```python
from build123d import *

# Parameters (mm, degrees)
SKETCH1_W                    = 28.1256
SKETCH1_H                    = 33.5
SKETCH1_W_2                  = 15.5256
SKETCH1_H_2                  = 15
BASE_FLANGE2_DEPTH           = 0.8128
EDGE_FLANGE3_STRIP_W         = 4.7244
EDGE_FLANGE3_STRIP_H         = 0.8128
EDGE_FLANGE3_STRIP_CUT_DEPTH = 33.5
EDGE_FLANGE3_DEPTH           = 33.5
EDGE_FLANGE3_FLAT_DEPTH      = 0.8128
EDGE_FLANGE4_START           = 0.7366
EDGE_FLANGE4_DEPTH           = 56.7698
EDGE_FLANGE4_START_2         = 57.1
EDGE_FLANGE4_2_DEPTH         = 0.4064
EDGE_FLANGE4_3_DEPTH         = 56.3634
CUT_EXTRUDE1_REACH           = 94.079
SKETCH22_R                   = 2.05
CUT_EXTRUDE2_REACH           = 89.705
SKETCH23_W                   = 11.2634
SKETCH23_H                   = 10
CUT_EXTRUDE3_REACH           = 93.47


# Read off the part's stored shape, not the designer's step: Edge-Flange4
# Sheet-metal steps are written as plain solids
with BuildPart() as part:
    # Sketch1 → Base-Flange2 (new body)
    with BuildSketch(Plane.XY):
        Rectangle(SKETCH1_W, SKETCH1_H)
        with Locations((0, 0.59)):
            Rectangle(SKETCH1_W_2, SKETCH1_H_2, mode=Mode.SUBTRACT)
    extrude(amount=-BASE_FLANGE2_DEPTH)

    # Edge-Flange3 strip (across the edge) → Edge-Flange3 strip cut (cut)
    with BuildSketch(Plane(origin=(-14.0628, 16.75, 0), x_dir=(1, 0, 0), z_dir=(0, -1, 0))):
        with Locations((-0.8128, -0.4064)):
            Rectangle(EDGE_FLANGE3_STRIP_W, EDGE_FLANGE3_STRIP_H)
    extrude(amount=EDGE_FLANGE3_STRIP_CUT_DEPTH, mode=Mode.SUBTRACT)

    # Edge-Flange3 bend section (across the edge) → Edge-Flange3 (add)
    with BuildSketch(Plane(origin=(-14.0628, 16.75, 0), x_dir=(1, 0, 0), z_dir=(0, -1, 0))):
        with BuildLine():
            Line((0, 0.7366), (0.8128, 0.7366))
            ThreePointArc((0.8128, 0.7366), (1.028545145, 0.215745145), (1.5494, 0))
            Line((1.5494, 0), (1.5494, -0.8128))
            ThreePointArc((1.5494, -0.8128), (0.453808753, -0.358991247), (0, 0.7366))
        make_face()
    extrude(amount=EDGE_FLANGE3_DEPTH)

    # Edge-Flange3 profile (on flange) → Edge-Flange3 flat (add)
    with BuildSketch(Plane(origin=(-14.0628, 0, 0), x_dir=(0, -1, 0), z_dir=(-1, 0, 0))):
        Polygon((-16.75, 0.7366), (16.75, 0.7366), (16.75, 57.1), (41.75, 57.1), (41.75, 77.1), (-16.75, 77.1), align=None)
    extrude(amount=-EDGE_FLANGE3_FLAT_DEPTH)

    # Edge-Flange4 outline → Edge-Flange4 (cut)
    with BuildSketch(Plane.XY.offset(EDGE_FLANGE4_START)):
        with BuildLine():
            ThreePointArc((-13.25, -15.2006), (-13.468624211, -15.994121367), (-14.0628, -16.563707039))
            Line((-14.0628, -16.563707039), (-14.0628, -16.75))
            Line((-14.0628, -16.75), (-13.25, -16.75))
            Line((-13.25, -16.75), (-13.25, -15.2006))
        make_face()
    extrude(amount=EDGE_FLANGE4_DEPTH, mode=Mode.SUBTRACT)

    # Edge-Flange4 2 outline → Edge-Flange4 2 (cut)
    with BuildSketch(Plane.XY.offset(EDGE_FLANGE4_START_2)):
        with BuildLine():
            Line((-14.0628, -14.7942), (-14.0628, -16.563707039))
            ThreePointArc((-14.0628, -16.563707039), (-13.468624211, -15.994121367), (-13.25, -15.2006))
            Line((-13.25, -15.2006), (-13.25, -14.7942))
            Line((-13.25, -14.7942), (-14.0628, -14.7942))
        make_face()
    extrude(amount=EDGE_FLANGE4_2_DEPTH, mode=Mode.SUBTRACT)

    # Edge-Flange4 3 outline → Edge-Flange4 3 (add)
    with BuildSketch(Plane.XY.offset(EDGE_FLANGE4_START)):
        with BuildLine():
            Line((-26.0628, -16.75), (-14.7994, -16.75))
            ThreePointArc((-14.7994, -16.75), (-14.419503755, -16.702704924), (-14.0628, -16.563707039))
            Line((-14.0628, -16.563707039), (-14.0628, -15.2006))
            ThreePointArc((-14.0628, -15.2006), (-14.278545145, -15.721454855), (-14.7994, -15.9372))
            Line((-14.7994, -15.9372), (-26.0628, -15.9372))
            Line((-26.0628, -15.9372), (-26.0628, -16.75))
        make_face()
    extrude(amount=EDGE_FLANGE4_3_DEPTH)

    # Sketch22 → Cut-Extrude1 (cut, up to next)
    with BuildSketch(Plane.ZY.offset(14.0628), mode=Mode.PRIVATE) as cut_extrude1_sk1:
        with Locations((67.1, -31.91)):
            Circle(SKETCH22_R)
    cut_extrude1_tool1 = extrude(cut_extrude1_sk1.sketch, amount=-CUT_EXTRUDE1_REACH, mode=Mode.PRIVATE) & part.part
    # Sketch22 → Cut-Extrude1 (cut, up to next)
    with BuildSketch(Plane.ZY.offset(14.0628), mode=Mode.PRIVATE) as cut_extrude1_sk2:
        with Locations((67.1, -9.41)):
            Circle(SKETCH22_R)
    cut_extrude1_tool2 = extrude(cut_extrude1_sk2.sketch, amount=-CUT_EXTRUDE1_REACH, mode=Mode.PRIVATE) & part.part
    # Sketch22 → Cut-Extrude1 (cut, up to next)
    with BuildSketch(Plane.ZY.offset(14.0628), mode=Mode.PRIVATE) as cut_extrude1_sk3:
        with Locations((49.895058849, 0.59)):
            Circle(SKETCH22_R)
    cut_extrude1_tool3 = extrude(cut_extrude1_sk3.sketch, amount=-CUT_EXTRUDE1_REACH, mode=Mode.PRIVATE) & part.part
    # Sketch22 → Cut-Extrude1 (cut, up to next)
    with BuildSketch(Plane.ZY.offset(14.0628), mode=Mode.PRIVATE) as cut_extrude1_sk4:
        with Locations((29.995058849, 0.59)):
            Circle(SKETCH22_R)
    cut_extrude1_tool4 = extrude(cut_extrude1_sk4.sketch, amount=-CUT_EXTRUDE1_REACH, mode=Mode.PRIVATE) & part.part
    # Sketch22 → Cut-Extrude1 (cut, up to next)
    with BuildSketch(Plane.ZY.offset(14.0628), mode=Mode.PRIVATE) as cut_extrude1_sk5:
        with Locations((10.095058849, 0.59)):
            Circle(SKETCH22_R)
    cut_extrude1_tool5 = extrude(cut_extrude1_sk5.sketch, amount=-CUT_EXTRUDE1_REACH, mode=Mode.PRIVATE) & part.part
    add(cut_extrude1_tool1.solids().sort_by_distance((-14.0628, -31.91, 67.1))[0], mode=Mode.SUBTRACT)
    add(cut_extrude1_tool2.solids().sort_by_distance((-14.0628, -9.41, 67.1))[0], mode=Mode.SUBTRACT)
    add(cut_extrude1_tool3.solids().sort_by_distance((-14.0628, 0.59, 49.895059))[0], mode=Mode.SUBTRACT)
    add(cut_extrude1_tool4.solids().sort_by_distance((-14.0628, 0.59, 29.995059))[0], mode=Mode.SUBTRACT)
    add(cut_extrude1_tool5.solids().sort_by_distance((-14.0628, 0.59, 10.095059))[0], mode=Mode.SUBTRACT)

    # Sketch23 → Cut-Extrude2 (cut, up to next)
    with BuildSketch(Plane(origin=(0, -15.9372, 0), x_dir=(1, 0, 0), z_dir=(0, 1, 0)), mode=Mode.PRIVATE) as cut_extrude2_sk1:
        with Locations((-20.4311, -29.2366)):
            Rectangle(SKETCH23_W, SKETCH23_H)
    cut_extrude2_tool1 = extrude(cut_extrude2_sk1.sketch, amount=-CUT_EXTRUDE2_REACH, mode=Mode.PRIVATE) & part.part
    # Sketch23 → Cut-Extrude2 (cut, up to next)
    with BuildSketch(Plane(origin=(0, -15.9372, 0), x_dir=(1, 0, 0), z_dir=(0, 1, 0)), mode=Mode.PRIVATE) as cut_extrude2_sk2:
        with BuildLine():
            Line((-22.8128, -18.4866), (-22.8128, -10.4866))
            ThreePointArc((-22.8128, -10.4866), (-20.0628, -7.7366), (-17.3128, -10.4866))
            Line((-17.3128, -10.4866), (-17.3128, -18.4866))
            ThreePointArc((-17.3128, -18.4866), (-20.0628, -21.2366), (-22.8128, -18.4866))
        make_face()
    cut_extrude2_tool2 = extrude(cut_extrude2_sk2.sketch, amount=-CUT_EXTRUDE2_REACH, mode=Mode.PRIVATE) & part.part
    # Sketch23 → Cut-Extrude2 (cut, up to next)
    with BuildSketch(Plane(origin=(0, -15.9372, 0), x_dir=(1, 0, 0), z_dir=(0, 1, 0)), mode=Mode.PRIVATE) as cut_extrude2_sk3:
        with BuildLine():
            Line((-22.8128, -39.9866), (-22.8128, -47.9866))
            ThreePointArc((-22.8128, -47.9866), (-20.0628, -50.7366), (-17.3128, -47.9866))
            Line((-17.3128, -47.9866), (-17.3128, -39.9866))
            ThreePointArc((-17.3128, -39.9866), (-20.0628, -37.2366), (-22.8128, -39.9866))
        make_face()
    cut_extrude2_tool3 = extrude(cut_extrude2_sk3.sketch, amount=-CUT_EXTRUDE2_REACH, mode=Mode.PRIVATE) & part.part
    add(cut_extrude2_tool1.solids().sort_by_distance((-20.4311, -15.9372, 29.2366))[0], mode=Mode.SUBTRACT)
    add(cut_extrude2_tool2.solids().sort_by_distance((-20.0628, -15.9372, 14.4866))[0], mode=Mode.SUBTRACT)
    add(cut_extrude2_tool3.solids().sort_by_distance((-20.0628, -15.9372, 43.9866))[0], mode=Mode.SUBTRACT)

    # Sketch26 → Cut-Extrude3 (cut, up to next)
    with BuildSketch(Plane.XY, mode=Mode.PRIVATE) as cut_extrude3_sk1:
        with BuildLine():
            Line((8.8128, -13.75), (10.3128, -13.75))
            ThreePointArc((10.3128, -13.75), (11.6128, -12.45), (10.3128, -11.15))
            Line((10.3128, -11.15), (8.8128, -11.15))
            ThreePointArc((8.8128, -11.15), (7.5128, -12.45), (8.8128, -13.75))
        make_face()
    cut_extrude3_tool1 = extrude(cut_extrude3_sk1.sketch, amount=-CUT_EXTRUDE3_REACH, mode=Mode.PRIVATE) & part.part
    # Sketch26 → Cut-Extrude3 (cut, up to next)
    with BuildSketch(Plane.XY, mode=Mode.PRIVATE) as cut_extrude3_sk2:
        with BuildLine():
            Line((-8.7634, -13.75), (-7.2634, -13.75))
            ThreePointArc((-7.2634, -13.75), (-5.9634, -12.45), (-7.2634, -11.15))
            Line((-7.2634, -11.15), (-8.7634, -11.15))
            ThreePointArc((-8.7634, -11.15), (-10.0634, -12.45), (-8.7634, -13.75))
        make_face()
    cut_extrude3_tool2 = extrude(cut_extrude3_sk2.sketch, amount=-CUT_EXTRUDE3_REACH, mode=Mode.PRIVATE) & part.part
    # Sketch26 → Cut-Extrude3 (cut, up to next)
    with BuildSketch(Plane.XY, mode=Mode.PRIVATE) as cut_extrude3_sk3:
        with BuildLine():
            Line((8.8128, 11.45), (10.3128, 11.45))
            ThreePointArc((10.3128, 11.45), (11.6128, 12.75), (10.3128, 14.05))
            Line((10.3128, 14.05), (8.8128, 14.05))
            ThreePointArc((8.8128, 14.05), (7.5128, 12.75), (8.8128, 11.45))
        make_face()
    cut_extrude3_tool3 = extrude(cut_extrude3_sk3.sketch, amount=-CUT_EXTRUDE3_REACH, mode=Mode.PRIVATE) & part.part
    # Sketch26 → Cut-Extrude3 (cut, up to next)
    with BuildSketch(Plane.XY, mode=Mode.PRIVATE) as cut_extrude3_sk4:
        with BuildLine():
            Line((-8.7634, 11.45), (-7.2634, 11.45))
            ThreePointArc((-7.2634, 11.45), (-5.9634, 12.75), (-7.2634, 14.05))
            Line((-7.2634, 14.05), (-8.7634, 14.05))
            ThreePointArc((-8.7634, 14.05), (-10.0634, 12.75), (-8.7634, 11.45))
        make_face()
    cut_extrude3_tool4 = extrude(cut_extrude3_sk4.sketch, amount=-CUT_EXTRUDE3_REACH, mode=Mode.PRIVATE) & part.part
    add(cut_extrude3_tool1.solids().sort_by_distance((9.5628, -12.45, 0))[0], mode=Mode.SUBTRACT)
    add(cut_extrude3_tool2.solids().sort_by_distance((-8.0134, -12.45, 0))[0], mode=Mode.SUBTRACT)
    add(cut_extrude3_tool3.solids().sort_by_distance((9.5628, 12.75, 0))[0], mode=Mode.SUBTRACT)
    add(cut_extrude3_tool4.solids().sort_by_distance((-8.0134, 12.75, 0))[0], mode=Mode.SUBTRACT)


solid = part.part
```
For this review, take the finished solid that the model builds, in its own axes (mm). A direction names the side the tool comes from. Coordinates: 2 decimals unless noted, no trailing zeros. Order: outer loops, then holes, each group sorted by start corner. A loop starts at its lowest first (then second) coordinate and runs counter-clockwise, first axis right, second up. Notation, with made-up numbers: (24, 0) -> (41, 0) arc R20 ccw to (41, 13) -> close; hole circle Ø8 at (-13.75, 34). An arc over 180 degrees is marked (long way). Use CSV: the item, a comma, the result in double quotes. Start each with the question number.
Item 1: We need section D-D, the plane z = 53.5. Give the boundary of the cut face in (x, y), then the cut area to 3 significant figures.
Item 2: Insertion check: pin 1 (9 mm diameter, centred on x = -23, z = 8.5, fed in from +Y); pin 2 (0.5 mm diameter, centred on x = -4.5, z = -0.5, fed in from -Y); pin 3 (0.7 mm diameter, centred on y = 1, z = -0.5, fed in from -X); pin 4 (12 mm diameter, centred on x = -3.5, z = 7, fed in from -Y). Each pin has a flat end and moves straight along its axis. Give the tip position at first contact, or say it passes through.
Item 3: We need section C-C, the plane z = 67.1. Give the boundary of the cut face in (x, y).
Item 4: For faces 1 (the face through (0.6, -7.2, -0.813)), 2 (the face through (-19.7, -16.2, 57.1)), 3 (the face through (-20.123, -16.338, 50.736)), 4 (the face through (-13.25, -6, 48)), 5 (the face through (-23, -15.937, 46)), list the 3-axis set-ups (+Z, -Z, +X, -X, +Y, -Y) from which the entire face can be reached by the end or side of a thin tool; tool diameter is ignored.
Item 5: We need section B-B, the plane x = -1.5. Give the boundary of the cut face in (y, z).
Item 6: Wall thickness on probe 1 along Y at (x, z) = (-13.9, 67.1); probe 2 along X at (y, z) = (-7, 57); probe 3 along Z at (x, y) = (10.5, 10.5): over which ranges is each line inside the solid? List them lowest first.
Item 7: We need section A-A, the plane y = -31.91. Give the boundary of the cut face in (x, z).
Item 8: Draft analysis for pull direction Y (two halves, no side actions). For faces 6 (the face through (-13.662, -0.195, 31.889)), 7 (the face through (-23, -15.937, 12)), 8 (the face through (0.6, -7.2, 0)), 9 (the face through (-23, -16.75, 46)), state which applies: pulls with the +Y half, pulls with the -Y half, needs draft (parallel to the pull), parting line crosses it, or undercut.
Derived:
1,outline,"(-26.06, -16.75) -> (-14.8, -16.75) arc R1.55 ccw to (-13.25, -15.2) -> (-13.25, 16.75) -> (-14.06, 16.75) -> (-14.06, -15.2) arc R0.74 cw to (-14.8, -15.94) -> (-26.06, -15.94) -> close"
1,area,"36.6 mm^2"
2,pin 1,"stops at y = -15.94"
2,pin 2,"stops at y = -16.75"
2,pin 3,"stops at x = -13.78"
2,pin 4,"passes through"
3,outline,"(-14.06, -41.75) -> (-13.25, -41.75) -> (-13.25, -33.96) -> (-14.06, -33.96) -> close; (-14.06, -29.86) -> (-13.25, -29.86) -> (-13.25, -11.46) -> (-14.06, -11.46) -> close; (-14.06, -7.36) -> (-13.25, -7.36) -> (-13.25, 16.75) -> (-14.06, 16.75) -> close"
4,face 1,"-Z, +X, -X, +Y, -Y"
4,face 2,"+X, -X"
4,face 3,"+Y, -Y"
4,face 4,"+Z, +X, +Y, -Y"
4,face 5,"+Z, -Z, -X, +Y"
5,outline,"(-16.75, -0.81) -> (-6.91, -0.81) -> (-6.91, 0) -> (-16.75, 0) -> close; (8.09, -0.81) -> (16.75, -0.81) -> (16.75, 0) -> (8.09, 0) -> close"
6,probe 1,"y = -41.75 to -33.96, -29.86 to -11.46, -7.36 to 16.75"
6,probe 2,"x = -14.06 to -13.25"
6,probe 3,"z = -0.81 to 0"
7,outline,"(-14.06, 57.1) -> (-13.25, 57.1) -> (-13.25, 65.05) -> (-14.06, 65.05) -> close; (-14.06, 69.15) -> (-13.25, 69.15) -> (-13.25, 77.1) -> (-14.06, 77.1) -> close"
8,face 6,"undercut"
8,face 7,"pulls with the +Y half"
8,face 8,"needs draft"
8,face 9,"pulls with the -Y half"
